from build123d import *

# Parameters (mm, degrees)
SKETCH_2_R      = 2.5
EXTRUDE_1_DEPTH = 3
FILLET_1_R      = 5


with BuildPart() as part:
    # ｽｹｯﾁ2 → ﾎﾞｽ - 押し出し1 (new body)
    with BuildSketch(Plane.XY):
        Polygon((10, 30), (30, 30), (30, 10), (10, 10), (10, -10), (-10, -10), (-10, 30), align=None)
        Circle(SKETCH_2_R, mode=Mode.SUBTRACT)
        with Locations((0, 20)):
            Circle(SKETCH_2_R, mode=Mode.SUBTRACT)
    extrude(amount=EXTRUDE_1_DEPTH)

    # ﾌｨﾚｯﾄ1
    fillet_1_edges = [part.edges().sort_by_distance(p)[0] for p in [
        (-10, 30, 1.5),
        (30, 30, 1.5),
        (30, 10, 1.5),
        (10, 10, 1.5),
        (10, -10, 1.5),
        (-10, -10, 1.5),
    ]]
    fillet(fillet_1_edges, radius=FILLET_1_R)


solid = part.part
Build history of the part. All positions in model axes, mm. A direction names the side the tool comes from. Give positions to 0.01 mm unless a question says otherwise; leave off trailing zeros. Order: outer loops, then holes, each group sorted by start corner. A loop starts at its lowest first (then second) coordinate and runs counter-clockwise, first axis right, second up. Notation, with made-up numbers: M 74.5,-29.5 L 132.5,-29.5 A19 ccw 132.5,-1.5 Z; hole C 87,34 d5. An arc over 180 degrees is marked long. Use one line per item in the form item = value.
1) Saw through at A-A (y = 20). Give the cut face in (x, z), plus the area to 3 significant figures.
Calculated:
outline = M -10,0 L -2.5,0 L -2.5,3 L -10,3 Z; M 2.5,0 L 30,0 L 30,3 L 2.5,3 Z
area = 105 mm2
2) Drop flat-ended pins along their axis: pin 1 (2 mm diameter, centred on x = 9, y = 1.5, fed in from -Z); pin 2 (1.5 mm diameter, centred on x = 18.5, z = 2, fed in from -Y). Give the stop position or say it passes through.
Calculated:
pin_1 = 0
pin_2 = 10
3) Saw through at D-D (y = 0). Give the cut face in (x, z), plus the area to 3 significant figures.
Calculated:
outline = M -10,0 L -2.5,0 L -2.5,3 L -10,3 Z; M 2.5,0 L 10,0 L 10,3 L 2.5,3 Z
area = 45.0 mm2
4) Probe probe 1 along Y at (x, z) = (0, 0.6); probe 2 along Y at (x, z) = (-1.5, 2.4); probe 3 along X at (y, z) = (18, 1.8). List the from-to ranges inside material, lowest first.
Calculated:
probe_1 = -10 to -2.5, 2.5 to 17.5, 22.5 to 30
probe_2 = -10 to -2, 2 to 18, 22 to 30
probe_3 = -10 to -1.5, 1.5 to 30
5) Saw through at C-C (x = 0). Give the cut face in (y, z), plus the area to 3 significant figures.
Calculated:
outline = M -10,0 L -2.5,0 L -2.5,3 L -10,3 Z; M 2.5,0 L 17.5,0 L 17.5,3 L 2.5,3 Z; M 22.5,0 L 30,0 L 30,3 L 22.5,3 Z
area = 90.0 mm2
6) Tool access for faces 4 (the face through (0, -10, 1)), 5 (the face through (20, 10, 1)): list every direction of +Z, -Z, +X, -X, +Y, -Y with a clear straight run to the whole face (end or side of a thin tool).
Calculated:
face_4 = +Z, -Z, +X, -X, -Y
face_5 = +Z, -Z, +X, -Y
7) Saw through at B-B (z = 1.45). Give the cut face in (x, y), plus the area to 3 significant figures.
Calculated:
outline = M -10,-5 A5 ccw -5,-10 L 5,-10 A5 ccw 10,-5 L 10,5 A5 cw 15,10 L 25,10 A5 ccw 30,15 L 30,25 A5 ccw 25,30 L -5,30 A5 ccw -10,25 Z; hole C 0,0 d5; hole C 0,20 d5
area = 1,140 mm2
8) Two-plate mould, pull along Y, no slides. Class faces 1 (the face through (10, 30, 1)), 2 (the face through (10, 0, 1)), 3 (the face through (-0.33, 22.48, 1.48)): released by +Y, released by -Y, zero draft, split by the parting line, or undercut.
Calculated:
face_1 = released by +Y
face_2 = zero draft
face_3 = undercut
